```python
from build123d import *

# Parameters (mm, degrees)
CUT_EXTRUDE1_START = -12
CUT_EXTRUDE1_DEPTH = 12
SKETCH3_R          = 2
CUT_EXTRUDE2_DEPTH = 4


with BuildPart() as part:
    # Sketch1 → Revolve1 (revolve)
    with BuildSketch(Plane.XY, mode=Mode.PRIVATE) as revolve1_sk:
        with BuildLine():
            ThreePointArc((21, 28.039082801), (19.960917199, 27), (21, 25.960917199))
            Line((21, 25.960917199), (21, 0))
            Line((21, 0), (0, 0))
            Line((0, 0), (0, 145))
            Line((0, 145), (4, 145))
            Line((4, 145), (4, 125))
            Line((4, 125), (12.5, 125))
            Line((12.5, 125), (12.5, 123))
            Line((12.5, 123), (21, 123))
            Line((21, 123), (21, 78))
            Line((21, 78), (19, 78))
            ThreePointArc((19, 78), (20.414213562, 77.414213562), (21, 76))
            Line((21, 76), (21, 75))
            Line((21, 75), (22.5, 75))
            Line((22.5, 75), (22.5, 35))
            Line((22.5, 35), (21, 35))
            Line((21, 35), (21, 28.039082801))
        make_face()
    revolve(revolve1_sk.sketch.rotate(Axis((0, 180.020988846, 0), (0, -1, 0)), 90), axis=Axis((0, 180.020988846, 0), (0, -1, 0)))

    # Sketch2 → Cut-Extrude1 (cut)
    with BuildSketch(Plane(origin=(0, 145, 0), x_dir=(1, 0, 0), z_dir=(0, 1, 0)).offset(CUT_EXTRUDE1_START)):
        with BuildLine():
            Line((-1.936491673, 3.5), (1.936491673, 3.5))
            ThreePointArc((1.936491673, 3.5), (0, 4), (-1.936491673, 3.5))
        make_face()
    extrude(amount=CUT_EXTRUDE1_DEPTH, mode=Mode.SUBTRACT)

    # Sketch3 → Cut-Extrude2 (cut)
    with BuildSketch(Plane(origin=(0, 123, 0), x_dir=(1, 0, 0), z_dir=(0, 1, 0))):
        with Locations(Location((0, 17.5, 0), (0, 0, 270))):
            Circle(SKETCH3_R)
        with Locations(Location((17.5, 0, 0), (0, 0, 270))):
            Circle(SKETCH3_R)
        with Locations(Location((0, -17.5, 0), (0, 0, 270))):
            Circle(SKETCH3_R)
        with Locations(Location((-17.5, 0, 0), (0, 0, 270))):
            Circle(SKETCH3_R)
    extrude(amount=-CUT_EXTRUDE2_DEPTH, mode=Mode.SUBTRACT)


solid = part.part
```
Geometry check sheet. Reference: the model listing, model coordinates, mm. A direction names the side the tool comes from. Coordinates: 2 decimals unless noted, no trailing zeros. Loops run counter-clockwise (first coordinate to the right, second up) from the corner with the lowest first, then second, coordinate; pieces in that order, holes last.
Item 1: Sectioned sample at A-A, the plane y = 131. Record the boundary of the cut face in (x, z), then the cut area to 3 significant figures.
Item 2: Go/stop test with flat-tipped pins: pin 1 Ø6 at (x, y) = (8.5, 65.5) entering from +Z; pin 2 Ø3 at (x, z) = (-0.5, 18.5) entering from +Y; pin 3 Ø1.2 at (x, z) = (0.5, -18) entering from +Y. Record where each tip stops, or that it passes through.
Item 3: Sectioned sample at B-B, the plane y = 13. Record the boundary of the cut face in (x, z).
Item 4: Thickness scan on line 1 (X direction, y = 121.55, z = 0); line 2 (Y direction, x = -6.5, z = -8.5); line 3 (Y direction, x = -10, z = -14). Record the ranges inside material, lowest first.
Item 5: Access from +Z, -Z, +X, -X, +Y, -Y to the whole of each face (thin tool, end or side, straight path). Record for faces 5 (the face through (20, 35, -7)), 6 (the face through (0, 145, 0)), 7 (the face through (-6.31, 75.49, 20.03)).
Item 6: Release check for a two-part mould opening along X. For faces 1 (the face through (-17, 119, 0)), 2 (the face through (-3.755, 123.986, 11.923)), 3 (the face through (-15.517, 121.028, -0.26)), 4 (the face through (0, 139, -3.5)) record: released by +X, released by -X, zero draft, split by the parting line, or undercut.
Check result:
1. outline: circle Ø8 at (0, 0)
1. area: 50.3 mm2
2. pin 1: stops at z = 21.82
2. pin 2: stops at y = 123
2. pin 3: stops at y = 119
3. outline: circle Ø42 at (0, 0)
4. line 1: x = -21 to -19.5, -15.5 to 15.5, 19.5 to 21
4. line 2: y = 0 to 125
4. line 3: y = 0 to 123
5. face 5: -Y
5. face 6: +Z, -Z, +X, -X, +Y
5. face 7: +Y
6. face 1: undercut
6. face 2: split by the parting line
6. face 3: undercut
6. face 4: zero draft
